Can you work these out from the model? Positions are in its coordinate system, mm. A direction names the side the tool comes from. Give positions to 0.01 mm unless a question says otherwise; leave off trailing zeros. Order: outer loops, then holes, each group sorted by start corner. A loop starts at its lowest first (then second) coordinate and runs counter-clockwise, first axis right, second up. Notation, with made-up numbers: M -17,17.25 L 38,17.25 A24 cw 38,27.25 Z; hole C 0.25,-9.75 d10. An arc over 180 degrees is marked long. Answer as a JSON object with one key per item and string values.
```python
from build123d import *

# Parameters (mm, degrees)
F0_W     = 80
F0_H     = 50
F1_DEPTH = 20
F2_W     = 100
F2_H     = 30
F3_DEPTH = 10
F4_W     = 40
F4_H     = 30
F5_DEPTH = 90
F6_SIZE2 = 19.99999
F6_SIZE  = 29.99999
F9_DEPTH = 50.001


# Not quite as in the source:
# - a fillet or chamfer is up to 0.001 mm smaller than in the source, because OpenCascade refuses the exact size


with BuildPart() as f1:
    # F0 (on Top) → F1 (new body)
    with BuildSketch(Plane.XY):
        with Locations((40, 25)):
            Rectangle(F0_W, F0_H)
    extrude(amount=F1_DEPTH)

    # F2 (on Top) → F3 (join)
    with BuildSketch(Plane.XY):
        with Locations((50, 65)):
            Rectangle(F2_W, F2_H)
    extrude(amount=F3_DEPTH)

    # F4 (on face) → F5 (join)
    with BuildSketch(Plane.XY.offset(10)):
        with Locations((20, 65)):
            Rectangle(F4_W, F4_H)
    extrude(amount=F5_DEPTH)

    # F6 (size 30 and 20 in the source; OpenCascade refuses exactly that, so slightly less here)
    f6_edges = [f1.edges().sort_by_distance(p)[0] for p in [
        (20, 50, 100),
    ]]
    f6_side = f1.faces().sort_by_distance((20, 65, 100))[0]
    chamfer(f6_edges, length=F6_SIZE, length2=F6_SIZE2, reference=f6_side)

    # F8 (on offset) → F9 (cut, through all)
    with BuildSketch(Plane(origin=(0, 0, 50), x_dir=(1, 0, 0), z_dir=(0, 0, -1))):
        with BuildLine():
            Line((30, -65), (40, -65))
            Line((40, -65), (40, -50))
            Line((40, -50), (20, -50))
            Line((20, -50), (20, -55))
            ThreePointArc((20, -55), (22.9289321881, -62.0710678119), (30, -65))
        make_face()
    extrude(amount=-F9_DEPTH, mode=Mode.SUBTRACT)


solid = f1.part
```
1) I want a section at B-B on z = 64.5. Write out the boundary of the cut face in (x, y), and give its area (3 significant figures).
Results found:
{"outline": "M 0,50 L 20,50 L 20,55 A10 cw 30,65 L 40,65 L 40,80 L 0,80 Z", "area": "921 mm²"}
2) I'm going to push flat-ended pins straight in: pin 1 Ø7.5 at (x, y) = (27, 59) entering from +Z; pin 2 Ø12 at (y, z) = (61, 59.5) entering from +X; pin 3 Ø1.5 at (y, z) = (53.5, 65) entering from +X. Where does each tip first touch, or does it pass through?
Results found:
{"pin 1": "stops at z = 50", "pin 2": "stops at x = 40", "pin 3": "stops at x = 20"}
3) I need wall thicknesses on L1, parallel to Z at x = 86, y = 74.5; L2, parallel to X at y = 71.5, z = 44.5; L3, parallel to X at y = 27, z = 9. Which ranges of each line are inside material? Lowest first, please.
Results found:
{"L1": "z = 0 to 10", "L2": "x = 0 to 40", "L3": "x = 0 to 80"}
4) For faces 1 (the face through (80, 25, 10)), 2 (the face through (40, 68, 44)), 3 (the face through (22.85, 61.99, 69.72)), which set-ups out of +Z, -Z, +X, -X, +Y, -Y let a thin tool reach every point of the face, with its end or its side?
Results found:
{"face 1": "+Z, -Z, +X, -Y", "face 2": "+Z, +X, +Y", "face 3": "+Z, +X, -Y"}
5) I want a section at C-C on y = 68. Write out the boundary of the cut face in (x, z).
Results found:
{"outline": "M 0,0 L 100,0 L 100,10 L 40,10 L 40,92 L 0,92 Z"}
